Design review of the part built by this model. Coordinates are the model's own, in mm. A direction names the side the tool comes from. Coordinates: 2 decimals unless noted, no trailing zeros. Write each loop counter-clockwise with the first axis right and the second up, starting at its lowest first coordinate (ties: lowest second). Pieces come first, ordered by that corner, then holes. Notation, with made-up numbers: M 3.5,23.5 L 14.5,23.5 A15 cw 14.5,34.5 Z; hole C 3.5,12 d7. An arc over 180 degrees is marked long. One line per question, with ' | ' between items.
from build123d import *

# Parameters (mm, degrees)
BOSS_EXTRUDE1_DEPTH = 62.5
BOSS_EXTRUDE2_DEPTH = 28
CUT_EXTRUDE1_DEPTH  = 76.805672611
SKETCH5_R           = 10
BOSS_EXTRUDE3_DEPTH = 20
HOLE1_D             = 9
HOLE1_DEPTH         = 16
BOSS_EXTRUDE5_START = -10
BOSS_EXTRUDE5_DEPTH = 2


with BuildPart() as part:
    # Sketch1 → Boss-Extrude1 (new body)
    with BuildSketch(Plane(origin=(0, 0, 0), x_dir=(0, 0, -1), z_dir=(1, 0, 0))):
        Polygon((-14, 16), (-14, 11), (-20, 11), (-20, 22), (0, 22), (0, -22), (-20, -22), (-20, -11), (-14, -11), (-14, -16), (-6, -16), (-6, 16), align=None)
    extrude(amount=BOSS_EXTRUDE1_DEPTH)

    # Sketch3 → Boss-Extrude2 (add)
    with BuildSketch(Plane.XY.offset(20)):
        with BuildLine():
            Line((12.5, 20), (12.5, -20))
            ThreePointArc((12.5, -20), (0, -32.5), (-12.5, -20))
            Line((-12.5, -20), (-12.5, 20))
            ThreePointArc((-12.5, 20), (0, 32.5), (12.5, 20))
        make_face()
    extrude(amount=-BOSS_EXTRUDE2_DEPTH)

    # Sketch4 → Cut-Extrude1 (cut, through all)
    with BuildSketch(Plane.XY.offset(20)):
        with BuildLine():
            Line((6.25, 20), (6.25, -20))
            ThreePointArc((6.25, -20), (0, -26.25), (-6.25, -20))
            Line((-6.25, -20), (-6.25, 20))
            ThreePointArc((-6.25, 20), (0, 26.25), (6.25, 20))
        make_face()
    extrude(amount=-CUT_EXTRUDE1_DEPTH, mode=Mode.SUBTRACT)

    # Sketch5 → Boss-Extrude3 (add)
    with BuildSketch(Plane(origin=(0, 22, 0), x_dir=(1, 0, 0), z_dir=(0, 1, 0))):
        with Locations(Location((37.5, -10, 0), (0, 0, 270))):
            Circle(SKETCH5_R)
    extrude(amount=BOSS_EXTRUDE3_DEPTH)

    # Hole1
    with Locations(Plane(origin=(0, 42, 0), x_dir=(1, 0, 0), z_dir=(0, 1, 0))):
        with Locations((37.5, -10)):
            Hole(HOLE1_D / 2, depth=HOLE1_DEPTH)

    # Sketch9 → Boss-Extrude5 (add, symmetric)
    with BuildSketch(Plane.XY.offset(20).offset(BOSS_EXTRUDE5_START)):
        Polygon((47.5, 40), (62.5, 22), (47.5, 22), (46.5, 22), (46.5, 40), align=None)
    extrude(amount=BOSS_EXTRUDE5_DEPTH, both=True)


solid = part.part
1. To check wall thickness, follow line 1 along Y through (x, z) = (27.5, 11.25); line 2 along Y through (x, z) = (41.5, 15.5); line 3 along X through (y, z) = (1.5, 5.75). State the ranges of each line that lie inside material, in increasing order. Write a range as [from, to].
Answer sheet:
line 1: [-22, -16], [16, 22] | line 2: [-22, -11], [11, 42] | line 3: [-12.5, -6.25], [6.25, 62.5]
2. Take a section at C-C (y = -12). Write out the cut boundary in (x, z).
Answer sheet:
outline: M -12.5,-8 L -6.25,-8 L -6.25,20 L -12.5,20 Z; M 6.25,-8 L 12.5,-8 L 12.5,0 L 62.5,0 L 62.5,6 L 12.5,6 L 12.5,14 L 62.5,14 L 62.5,20 L 6.25,20 Z
3. Take a section at B-B (z = -1.75). Write out the cut boundary in (x, y).
Answer sheet:
outline: M -12.5,-20 A12.5 ccw 12.5,-20 L 12.5,20 A12.5 ccw -12.5,20 Z; hole M -6.25,-20 A6.25 ccw 6.25,-20 L 6.25,20 A6.25 ccw -6.25,20 Z
4. Draft analysis for pull direction Y (two halves, no side actions). For faces 1 (the face through (37, 0, 0)), 2 (the face through (37, -13, 14)), 3 (the face through (0.275, -32.497, 6.196)), state which applies: pulls with the +Y half, pulls with the -Y half, needs draft (parallel to the pull), parting line crosses it, or undercut.
Answer sheet:
face 1: needs draft | face 2: undercut | face 3: pulls with the -Y half
5. Take a section at D-D (x = 16). Write out the cut boundary in (y, z), then the cut area to 3 significant figures.
Answer sheet:
outline: M -22,0 L 22,0 L 22,20 L 11,20 L 11,14 L 16,14 L 16,6 L -16,6 L -16,14 L -11,14 L -11,20 L -22,20 Z | area: 492 mm^2
6. Take a section at A-A (x = 0). Write out the cut boundary in (y, z), then the cut area to 3 significant figures.
Answer sheet:
outline: M -32.5,-8 L -26.25,-8 L -26.25,20 L -32.5,20 Z; M 26.25,-8 L 32.5,-8 L 32.5,20 L 26.25,20 Z | area: 350 mm^2
7. Insertion check: pin 1 Ø5 at (x, z) = (12, 0) entering from -Y; pin 2 Ø1 at (x, z) = (25.5, 15) entering from +Y; pin 3 Ø4.5 at (x, y) = (52.5, 33.5) entering from +Z. Each pin has a flat end and moves straight along its axis. Give the tip position at first contact, or say it passes through.
Answer sheet:
pin 1: y = -28.12 | pin 2: y = 22 | pin 3: z = 12
8. Tool access review of faces 4 (the face through (37, -11, 17)), 5 (the face through (37, 0, 6)), 6 (the face through (12.5, 0, -4)), 7 (the face through (-6.25, 0, 6)): name each direction out of +Z, -Z, +X, -X, +Y, -Y from which nothing blocks a thin tool from reaching the whole face with its end or side.
Answer sheet:
face 4: +Z, +X | face 5: +X | face 6: -Z, +X, +Y, -Y | face 7: +Z, -Z
